Work out the finished part from the listing and answer in its coordinate system (mm). A direction names the side the tool comes from. Give positions to 0.01 mm unless a question says otherwise; leave off trailing zeros. Order: outer loops, then holes, each group sorted by start corner. A loop starts at its lowest first (then second) coordinate and runs counter-clockwise, first axis right, second up. Notation, with made-up numbers: (87, 89) -> (119, 89) arc R20 cw to (119, 121) -> close; hole circle Ø7 at (11, 2.25). An arc over 180 degrees is marked (long way). Answer as CSV lines item,"result". Start each with the question number.
1. A cutting plane is placed at A-A (x = -27). Give the vertices of the cut face in (y, z), then the cut area to 3 significant figures.
2. Find the intervals of material crossed by L1, parallel to X at y = -10.5, z = -451; L2, parallel to Y at x = -22, z = -755; L3, parallel to Y at x = -16, z = -395.5, in increasing order.
3. For faces 4 (the flat face through (-25, -38.5, -404)), 5 (the flat face through (-25, 0, -404)), determine the directions among +Z, -Z, +X, -X, +Y, -Y from which every point of the face is accessible in a straight line to the end or side of a thin tool.
4. For a pull along Y with two mould halves and no side action, classify faces 1 (the flat face through (-16.465, -20, -404)), 2 (the flat face through (-25, -40, -404)), 3 (the flat face through (-14.965, -20, -404)) as released by +Y, released by -Y, zero draft, split by the parting line, or undercut.
5. A cutting plane is placed at C-C (z = -152). Give the vertices of the cut face in (x, y), then the cut area to 3 significant figures.
6. A cutting plane is placed at B-B (y = -29.5). Give the vertices of the cut face in (x, z), then the cut area to 3 significant figures.
from build123d import *

# Parameters (mm, degrees)
EXTRUDE_START   = -410
EXTRUDE_1_DEPTH = 410


# Read off the part's stored shape, not the designer's step: Бобышка-Вытянуть1
with BuildPart() as part:
    # Бобышка-Вытянуть1 outline → Бобышка-Вытянуть1 (new body)
    with BuildSketch(Plane.XY.offset(EXTRUDE_START)):
        with BuildLine():
            ThreePointArc((-34.964986884, -38.5), (-34.525647056, -39.560660172), (-33.464986884, -40))
            Line((-33.464986884, -40), (-16.464986884, -40))
            ThreePointArc((-16.464986884, -40), (-15.404326712, -39.560660172), (-14.964986884, -38.5))
            Line((-14.964986884, -38.5), (-14.964986884, -1.5))
            ThreePointArc((-14.964986884, -1.5), (-15.404326712, -0.439339828), (-16.464986884, 0))
            Line((-16.464986884, 0), (-33.464986884, 0))
            ThreePointArc((-33.464986884, 0), (-34.525647056, -0.439339828), (-34.964986884, -1.5))
            Line((-34.964986884, -1.5), (-34.964986884, -38.5))
        make_face()
        with BuildLine():
            Line((-33.464986884, -37.5), (-33.464986884, -2.5))
            ThreePointArc((-33.464986884, -2.5), (-33.172093665, -1.792893219), (-32.464986884, -1.5))
            Line((-32.464986884, -1.5), (-17.464986884, -1.5))
            ThreePointArc((-17.464986884, -1.5), (-16.757880103, -1.792893219), (-16.464986884, -2.5))
            Line((-16.464986884, -2.5), (-16.464986884, -37.5))
            ThreePointArc((-16.464986884, -37.5), (-16.757880103, -38.207106781), (-17.464986884, -38.5))
            Line((-17.464986884, -38.5), (-32.464986884, -38.5))
            ThreePointArc((-32.464986884, -38.5), (-33.172093665, -38.207106781), (-33.464986884, -37.5))
        make_face(mode=Mode.SUBTRACT)
    extrude(amount=EXTRUDE_1_DEPTH)

    # Зеркальное отражение1: part across plane


with BuildPart() as part_1:
    add(part.part)
    add(part.part.mirror(Plane(origin=(441.299876816, -806.206552751, -410), x_dir=(1, 0, 0), z_dir=(0, 0, 1))))


solid = part_1.part
Answer sheet:
1,outline,"(-40, -820) -> (-38.5, -820) -> (-38.5, 0) -> (-40, 0) -> close; (-1.5, -820) -> (0, -820) -> (0, 0) -> (-1.5, 0) -> close"
1,area,"2,460 mm^2"
2,L1,"x = -34.96 to -33.46, -16.46 to -14.96"
2,L2,"y = -40 to -38.5, -1.5 to 0"
2,L3,"y = -39.93 to -0.07"
3,face 4,"+Z, -Z"
3,face 5,"+Z, -Z, +X, -X, +Y"
4,face 1,"undercut"
4,face 2,"released by -Y"
4,face 3,"zero draft"
5,outline,"(-34.96, -38.5) arc R1.5 ccw to (-33.46, -40) -> (-16.46, -40) arc R1.5 ccw to (-14.96, -38.5) -> (-14.96, -1.5) arc R1.5 ccw to (-16.46, 0) -> (-33.46, 0) arc R1.5 ccw to (-34.96, -1.5) -> close; hole (-33.46, -37.5) arc R1 ccw to (-32.46, -38.5) -> (-17.46, -38.5) arc R1 ccw to (-16.46, -37.5) -> (-16.46, -2.5) arc R1 ccw to (-17.46, -1.5) -> (-32.46, -1.5) arc R1 ccw to (-33.46, -2.5) -> close"
5,area,"170 mm^2"
6,outline,"(-34.96, -820) -> (-33.46, -820) -> (-33.46, 0) -> (-34.96, 0) -> close; (-16.46, -820) -> (-14.96, -820) -> (-14.96, 0) -> (-16.46, 0) -> close"
6,area,"2,460 mm^2"
